from build123d import *

# Parameters (mm, degrees)
F1_DEPTH = 5
F2_D     = 5.4
F3_W     = 3
F3_H     = 2
F4_DEPTH = 10
F5_R     = 1.49999


# Not quite as in the source:
# - a fillet or chamfer is up to 0.001 mm smaller than in the source, because OpenCascade refuses the exact size


with BuildPart() as f1:
    # F0 (on Top) → F1 (new body)
    with BuildSketch(Plane.XY):
        with BuildLine():
            ThreePointArc((-17.0389572543, 21.7029743907), (-15.8620482104, 20.0392796609), (-15.4467487052, 18.0441552605))
            Line((-15.4467487052, 18.0441552605), (-15.4467487052, -7.0029299584))
            Line((-15.4467487052, -7.0029299584), (-12.9467487052, -15.0029299584))
            Line((-12.9467487052, -15.0029299584), (-10.4467487052, -7.0029299584))
            Line((-10.4467487052, -7.0029299584), (-10.4467487052, 9.9970700416))
            ThreePointArc((-10.4467487052, 9.9970700416), (-8.9822826112, 13.5326039476), (-5.4467487052, 14.9970700416))
            Line((-5.4467487052, 14.9970700416), (0, 14.9970700416))
            Line((0, 14.9970700416), (0, 37.4970700416))
            ThreePointArc((0, 37.4970700416), (-2.5, 39.9970700416), (0, 42.4970700416))
            Line((0, 42.4970700416), (0, 64.9970700416))
            Line((0, 64.9970700416), (-5, 64.9970700416))
            Line((-5, 64.9970700416), (-9.6153846154, 63.0739931186))
            ThreePointArc((-9.6153846154, 63.0739931186), (-24.6069864626, 44.4125221395), (-17.0389572543, 21.7029743907))
        make_face()
        with BuildLine():
            Line((0, 37.4970700416), (0, 42.4970700416))
            ThreePointArc((0, 42.4970700416), (-2.5, 39.9970700416), (0, 37.4970700416))
        make_face()
        with BuildLine():
            Line((5, 64.9970700416), (0, 64.9970700416))
            Line((0, 64.9970700416), (0, 42.4970700416))
            ThreePointArc((0, 42.4970700416), (2.5, 39.9970700416), (0, 37.4970700416))
            Line((0, 37.4970700416), (0, 14.9970700416))
            Line((0, 14.9970700416), (5.4467487052, 14.9970700416))
            ThreePointArc((5.4467487052, 14.9970700416), (8.9822826112, 13.5326039476), (10.4467487052, 9.9970700416))
            Line((10.4467487052, 9.9970700416), (10.4467487052, -7.0029299584))
            Line((10.4467487052, -7.0029299584), (12.9467487052, -15.0029299584))
            Line((12.9467487052, -15.0029299584), (15.4467487052, -7.0029299584))
            Line((15.4467487052, -7.0029299584), (15.4467487052, 18.0441552605))
            ThreePointArc((15.4467487052, 18.0441552605), (15.8620482104, 20.0392796609), (17.0389572543, 21.7029743907))
            ThreePointArc((17.0389572543, 21.7029743907), (24.6069864626, 44.4125221395), (9.6153846154, 63.0739931186))
            Line((9.6153846154, 63.0739931186), (5, 64.9970700416))
        make_face()
        with BuildLine():
            ThreePointArc((0, 37.4970700416), (2.5, 39.9970700416), (0, 42.4970700416))
            Line((0, 42.4970700416), (0, 37.4970700416))
        make_face()
    extrude(amount=F1_DEPTH)

    # F2 (through all)
    with Locations(Plane(origin=(0, 0, 0), x_dir=(1, 0, 0), z_dir=(0, 0, -1))):
        with Locations((0, -39.9970700416)):
            Hole(F2_D / 2)

    # F3 (on face) → F4 (cut)
    with BuildSketch(Plane(origin=(0, 64.9970700416, 0), x_dir=(-1, 0, 0), z_dir=(0, 1, 0))):
        with Locations((0, 2.5)):
            Rectangle(F3_W, F3_H)
    extrude(amount=-F4_DEPTH, mode=Mode.SUBTRACT)

    # F5 (radius 1.5 in the source; OpenCascade refuses exactly that, so slightly less here)
    f5_edges = [f1.edges().sort_by_distance(p)[0] for p in [
        (1.5, 59.99707, 3.5),
        (-1.5, 59.99707, 3.5),
    ]]
    fillet(f5_edges, radius=F5_R)


solid = f1.part
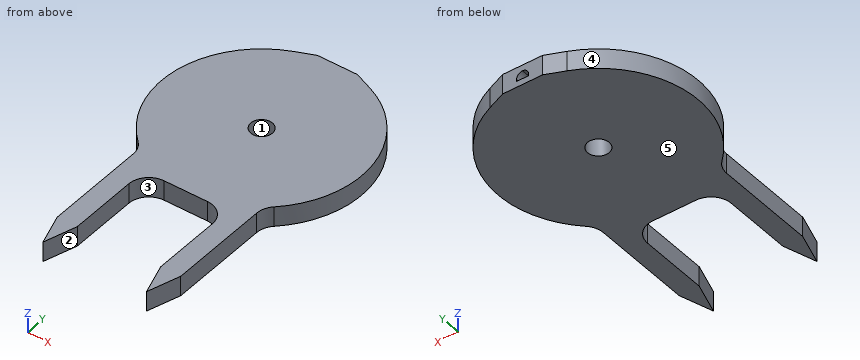
Geometry check sheet. Reference: the model listing, model coordinates, mm. Face numbers are marked on the shaded views. A direction names the side the tool comes from. Give positions to 0.01 mm unless a question says otherwise; leave off trailing zeros. Order: outer loops, then holes, each group sorted by start corner. A loop starts at its lowest first (then second) coordinate and runs counter-clockwise, first axis right, second up. Notation, with made-up numbers: (35.25, 70.25) - (83.25, 70.25) arc R11 cw to (83.25, 90.25) - close; hole circle Ø3 at (67.25, -34). An arc over 180 degrees is marked (long way). Answer as a JSON object with one key per item and string values.
(1) Draft check along X on the marked faces 3, 4 and 5. Enter one of: released by +X, released by -X, zero draft, split by the parting line, or undercut.
Report:
{"face 3": "undercut", "face 4": "released by -X", "face 5": "zero draft"}
(2) Tool access check on the marked faces 1 and 2. Record the directions out of +Z, -Z, +X, -X, +Y, -Y that give a thin tool (end or side, any length) a straight path to the whole face; none if there is none.
Report:
{"face 1": "+Z, -Z", "face 2": "+Z, -Z, -Y"}
(3) Material ranges on line 1 (X direction, y = 0, z = 2.6); line 2 (Y direction, x = 0, z = 3.4); line 3 (Y direction, x = 0, z = 1.1), recorded low to high.
Report:
{"line 1": "-15.45 to -10.45, 10.45 to 15.45", "line 2": "15 to 37.3, 42.7 to 55", "line 3": "15 to 37.3, 42.7 to 65"}
(4) Cross-section at A-A (y = 13). Record the cut outline in (x, z).
Report:
{"outline": "(-15.45, 0) - (-9.44, 0) - (-9.44, 5) - (-15.45, 5) - close; (9.44, 0) - (15.45, 0) - (15.45, 5) - (9.44, 5) - close"}
(5) Cross-section at C-C (x = 19). Record the cut outline in (y, z), then the cut area to 3 significant figures.
Report:
{"outline": "(23.75, 0) - (56.25, 0) - (56.25, 5) - (23.75, 5) - close", "area": "162 mm^2"}
(6) Cross-section at D-D (y = 25.5). Record the cut outline in (x, z).
Report:
{"outline": "(-20.37, 0) - (20.37, 0) - (20.37, 5) - (-20.37, 5) - close"}
(7) Depth check by flat-ended pin: pin 1 Ø1.5 at (y, z) = (0, 2.5) entering from +X; pin 2 Ø1 at (x, y) = (19.5, 22) entering from -Z; pin 3 Ø3 at (x, z) = (-14.5, 1) entering from +Y; pin 4 Ø1.5 at (x, z) = (6, 1.5) entering from +Y. Enter the tip coordinate at first touch or a pass-through.
Report:
{"pin 1": "x = 15.45", "pin 2": "through", "pin 3": "y = 61.35", "pin 4": "y = 64.89"}
